For this review, take the finished solid that the model builds, in its own axes (mm). A direction names the side the tool comes from. Round coordinates to 2 decimals unless told otherwise and drop trailing zeros. Write each loop counter-clockwise with the first axis right and the second up, starting at its lowest first coordinate (ties: lowest second). Pieces come first, ordered by that corner, then holes.
from build123d import *

# Parameters (mm, degrees)
SKETCH1_R           = 7.975
SKETCH1_R_2         = 1.25
BOSS_EXTRUDE1_DEPTH = 6.35


with BuildPart() as part:
    # Sketch1 → Boss-Extrude1 (new body)
    with BuildSketch(Plane(origin=(0, 0, 0), x_dir=(1, 0, 0), z_dir=(0, 1, 0))):
        with BuildLine():
            Line((13.53608603, 7.5), (100, 7.5))
            Line((100, 7.5), (100, -7.5))
            Line((100, -7.5), (13.53608603, -7.5))
            ThreePointArc((13.53608603, -7.5), (-15.475, 0), (13.53608603, 7.5))
        make_face()
        with Locations(Location((0, 0, 0), (0, 0, 270))):
            Circle(SKETCH1_R, mode=Mode.SUBTRACT)
        with Locations(Location((0, -11.725, 0), (0, 0, 270))):
            Circle(SKETCH1_R_2, mode=Mode.SUBTRACT)
        with Locations(Location((0, 11.725, 0), (0, 0, 270))):
            Circle(SKETCH1_R_2, mode=Mode.SUBTRACT)
        with BuildLine():
            Line((55, 2.05), (95, 2.05))
            ThreePointArc((95, 2.05), (97.05, 0), (95, -2.05))
            Line((95, -2.05), (55, -2.05))
            ThreePointArc((55, -2.05), (52.95, 0), (55, 2.05))
        make_face(mode=Mode.SUBTRACT)
    extrude(amount=BOSS_EXTRUDE1_DEPTH)


solid = part.part
(1) For faces 4 (the face through (97.05, 3.13, -0.05)), 5 (the face through (56, 3, -7.5)), 6 (the face through (57, 3, 7.5)), list the 3-axis set-ups (+Z, -Z, +X, -X, +Y, -Y) from which the entire face can be reached by the end or side of a thin tool; tool diameter is ignored.
Geometry check:
face 4: +Y, -Y
face 5: -Z, +X, +Y, -Y
face 6: +Z, +X, +Y, -Y
(2) For line 1 along Z through (x, y) = (76, 4.5); line 2 along Z through (x, y) = (54, 4); line 3 along X through (y, z) = (6.25, -6), list the stretches that pass through material, from the lowest coordinate up.
Geometry check:
line 1: z = -7.5 to -2.05, 2.05 to 7.5
line 2: z = -7.5 to -1.79, 1.79 to 7.5
line 3: x = -14.26 to -5.25, 5.25 to 100
(3) We need section D-D, the plane z = 0. Give the boundary of the cut face in (x, y) (3 decimals), and give its area (3 significant figures).
Geometry check:
outline: (-15.475, 0) - (-7.975, 0) - (-7.975, 6.35) - (-15.475, 6.35) - close; (7.975, 0) - (52.95, 0) - (52.95, 6.35) - (7.975, 6.35) - close; (97.05, 0) - (100, 0) - (100, 6.35) - (97.05, 6.35) - close
area: 352 mm2
(4) We need section C-C, the plane y = 3.25. Give the boundary of the cut face in (x, z) (3 decimals).
Geometry check:
outline: (13.536, -7.5) - (100, -7.5) - (100, 7.5) - (13.536, 7.5) arc R15.475 ccw (long way) to start; hole circle Ø15.95 at (0, 0); hole circle Ø2.5 at (0, -11.725); hole circle Ø2.5 at (0, 11.725); hole (55, -2.05) - (95, -2.05) arc R2.05 ccw to (95, 2.05) - (55, 2.05) arc R2.05 ccw to start
(5) Mouldability with a two-part tool opening along X and no side actions: class faces 1 (the face through (2.395, 3.131, 7.607)), 2 (the face through (43, 0, 0)), 3 (the face through (-15.464, 3.131, 0.571)) as pulls with the +X half, pulls with the -X half, needs draft (parallel to the pull), parting line crosses it, or undercut.
Geometry check:
face 1: undercut
face 2: needs draft
face 3: parting line crosses it
(6) We need section B-B, the plane x = 79. Give the boundary of the cut face in (y, z).
Geometry check:
outline: (0, -7.5) - (6.35, -7.5) - (6.35, -2.05) - (0, -2.05) - close; (0, 2.05) - (6.35, 2.05) - (6.35, 7.5) - (0, 7.5) - close
(7) For pin 1 Ø3 at (x, y) = (70.5, 4) entering from +Z; pin 2 Ø3 at (x, y) = (68.5, 2.5) entering from -Z; pin 3 Ø3 at (y, z) = (1.5, 4) entering from -X, all flat-tipped, find the tip position at first contact; note any pin that passes through.
Geometry check:
pin 1: stops at z = 7.5
pin 2: stops at z = -7.5
pin 3: stops at x = -15.27
(8) We need section A-A, the plane x = 0. Give the boundary of the cut face in (y, z) (3 decimals).
Geometry check:
outline: (0, -15.475) - (6.35, -15.475) - (6.35, -12.975) - (0, -12.975) - close; (0, -10.475) - (6.35, -10.475) - (6.35, -7.975) - (0, -7.975) - close; (0, 7.975) - (6.35, 7.975) - (6.35, 10.475) - (0, 10.475) - close; (0, 12.975) - (6.35, 12.975) - (6.35, 15.475) - (0, 15.475) - close
